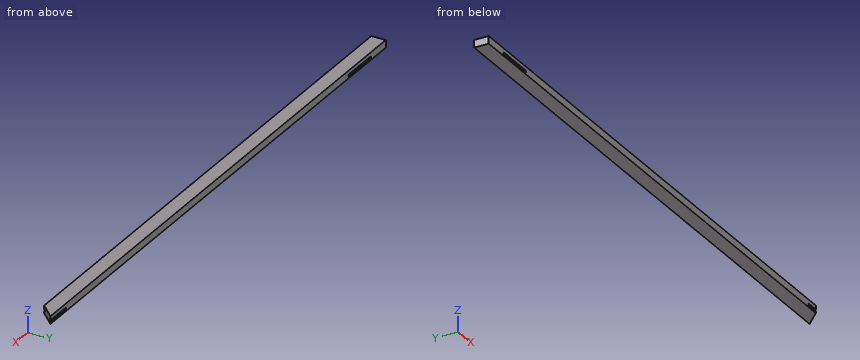
```python
from build123d import *

# Parameters (mm, degrees)
EXTRUDE_1_DEPTH     = 25
SKETCH_2_W          = 115
SKETCH_2_H          = 6
CUT_EXTRUDE_1_DEPTH = 7.5
DRAFT_1_ANGLE       = 45
MIRROR_START        = 6
MIRROR_1_DEPTH      = 6
CUT_EXTRUDE_START   = -13
CUT_EXTRUDE_2_DEPTH = 6


# Read off the part's stored shape, not the designer's step: 镜向1
with BuildPart() as part:
    # 草图1 → 凸台-拉伸1 (new body)
    with BuildSketch(Plane.XY):
        Polygon((0, 24), (1922, 24), (1874, -24), (0, -24), align=None)
    extrude(amount=EXTRUDE_1_DEPTH)

    # 草图2 → 切除-拉伸1 (cut)
    with BuildSketch(Plane.XZ.offset(24)):
        with Locations((149, 9)):
            Rectangle(SKETCH_2_W, SKETCH_2_H)
    extrude(amount=-CUT_EXTRUDE_1_DEPTH, mode=Mode.SUBTRACT)

    # 拔模1
    draft_1_faces = [part.faces().sort_by_distance(p)[0] for p in [
        (206.5, -20.25, 9),
        (91.5, -20.25, 9),
    ]]
    draft(draft_1_faces, Plane(origin=(0, -16.5, 0), x_dir=(-1, 0, 0), z_dir=(0, -1, 0)), DRAFT_1_ANGLE)

    # 镜向1 outline → 镜向1 (cut)
    with BuildSketch(Plane.XY.offset(MIRROR_START)):
        Polygon((84, 24), (91.5, 16.5), (206.5, 16.5), (214, 24), align=None)
    extrude(amount=MIRROR_1_DEPTH, mode=Mode.SUBTRACT)

    # 草图3 → 切除-拉伸2 (cut)
    with BuildSketch(Plane.XY.offset(25).offset(CUT_EXTRUDE_START)):
        Polygon((1832.5, 24), (1840, 16.5), (1914.5, 16.5), (1922, 24), align=None)
        Polygon((1832.5, -24), (1840, -16.5), (1881.5, -16.5), (1874, -24), align=None)
    extrude(amount=-CUT_EXTRUDE_2_DEPTH, mode=Mode.SUBTRACT)


solid = part.part
```
Verification items for the finished model (mm, model axes). Coordinates: 2 decimals unless noted, no trailing zeros. Loops run counter-clockwise (first coordinate to the right, second up) from the corner with the lowest first, then second, coordinate; pieces in that order, holes last. Notation, with made-up numbers: (52.25, 84) - (69.25, 84) arc R29 ccw to (69.25, 105) - close; hole circle Ø11 at (-34, 89). An arc over 180 degrees is marked (long way). Put each result on its own line as item: value.
Item 1: Section check A-A (x = 168.5). Enter the section's corners in (y, z), then the cut area to 3 significant figures.
Conclusion:
outline: (-24, 0) - (24, 0) - (24, 6) - (16.5, 6) - (16.5, 12) - (24, 12) - (24, 25) - (-24, 25) - (-24, 12) - (-16.5, 12) - (-16.5, 6) - (-24, 6) - close
area: 1,110 mm2
Item 2: Section check B-B (y = -9). Enter the section's corners in (x, z).
Conclusion:
outline: (0, 0) - (1889, 0) - (1889, 25) - (0, 25) - close
Item 3: Scan lines: line 1 along X through (y, z) = (-20.5, 23.5); line 2 along X through (y, z) = (17.5, 17). Record each from-to range of solid material in increasing order.
Conclusion:
line 1: x = 0 to 1877.5
line 2: x = 0 to 1915.5
Item 4: Gauge pin test, flat ends, axial feed: pin 1 Ø3 at (x, z) = (1869, 9) entering from +Y; pin 2 Ø6 at (y, z) = (3, 20) entering from +X. Record the tip position at first contact, or that the pin passes through.
Conclusion:
pin 1: stops at y = 16.5
pin 2: stops at x = 1904
